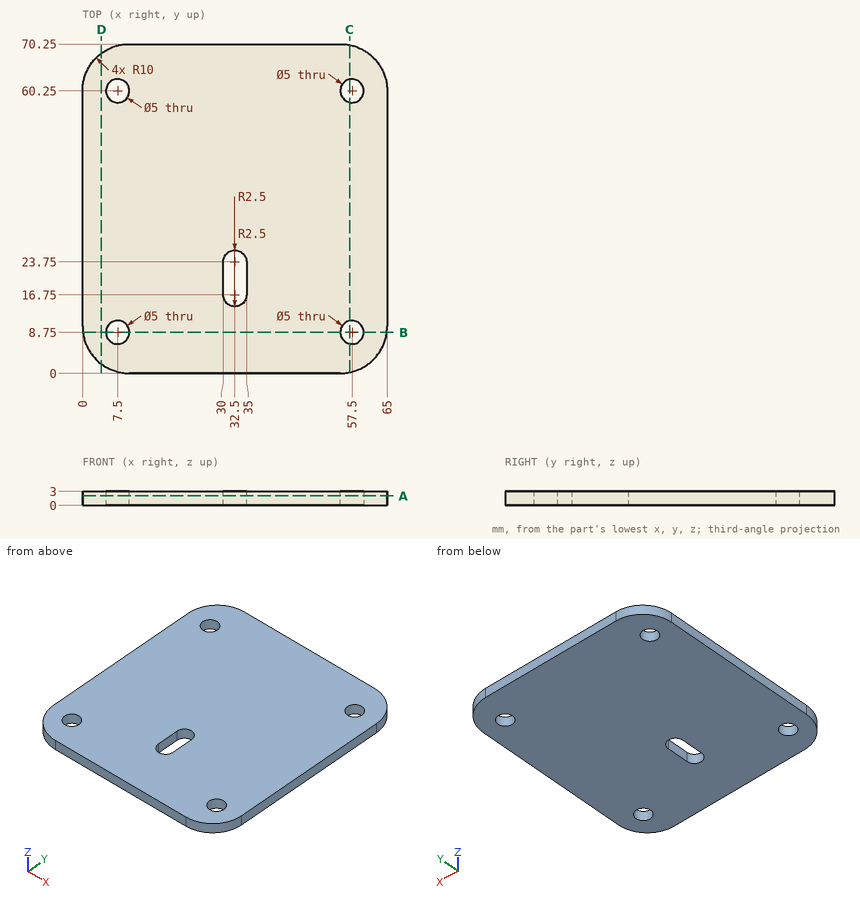
Design review of the part shown in the three views and the two pictorial views. Dimensions are in mm from the part's minimum x, y and z. Round coordinates to 2 decimals unless told otherwise and drop trailing zeros. Order: outer loops, then holes, each group sorted by start corner. A loop starts at its lowest first (then second) coordinate and runs counter-clockwise, first axis right, second up.
(1) Take a section at D-D, the plane x = 4. State the section outline as (y, z) points.
Working result:
outline: (2, 0) - (68.25, 0) - (68.25, 3) - (2, 3) - close
(2) Wall thickness on L1, parallel to Y at x = 57, z = 1.5; L2, parallel to X at y = 8, z = 0.65; L3, parallel to Y at x = 58.5, z = 1.35: over which ranges is each line inside the solid? List them lowest first.
Working result:
L1: y = 0.2 to 6.3, 11.2 to 57.8, 62.7 to 70.05
L2: x = 0.2 to 5.12, 9.88 to 55.12, 59.88 to 64.8
L3: y = 0.63 to 6.46, 11.04 to 57.96, 62.54 to 69.62
(3) Take a section at A-A, the plane z = 2. State the section outline as (x, y) points.
Working result:
outline: (0, 10) arc R10 ccw to (10, 0) - (55, 0) arc R10 ccw to (65, 10) - (65, 60.25) arc R10 ccw to (55, 70.25) - (10, 70.25) arc R10 ccw to (0, 60.25) - close; hole circle Ø5 at (7.5, 8.75); hole circle Ø5 at (7.5, 60.25); hole (30, 16.75) arc R2.5 ccw to (35, 16.75) - (35, 23.75) arc R2.5 ccw to (30, 23.75) - close; hole circle Ø5 at (57.5, 8.75); hole circle Ø5 at (57.5, 60.25)
(4) Take a section at C-C, the plane x = 57. State the section outline as (y, z) points, plus the area to 3 significant figures.
Working result:
outline: (0.2, 0) - (6.3, 0) - (6.3, 3) - (0.2, 3) - close; (11.2, 0) - (57.8, 0) - (57.8, 3) - (11.2, 3) - close; (62.7, 0) - (70.05, 0) - (70.05, 3) - (62.7, 3) - close
area: 180 mm2
(5) Take a section at B-B, the plane y = 8.75. State the section outline as (x, z) points.
Working result:
outline: (0.08, 0) - (5, 0) - (5, 3) - (0.08, 3) - close; (10, 0) - (55, 0) - (55, 3) - (10, 3) - close; (60, 0) - (64.92, 0) - (64.92, 3) - (60, 3) - close
